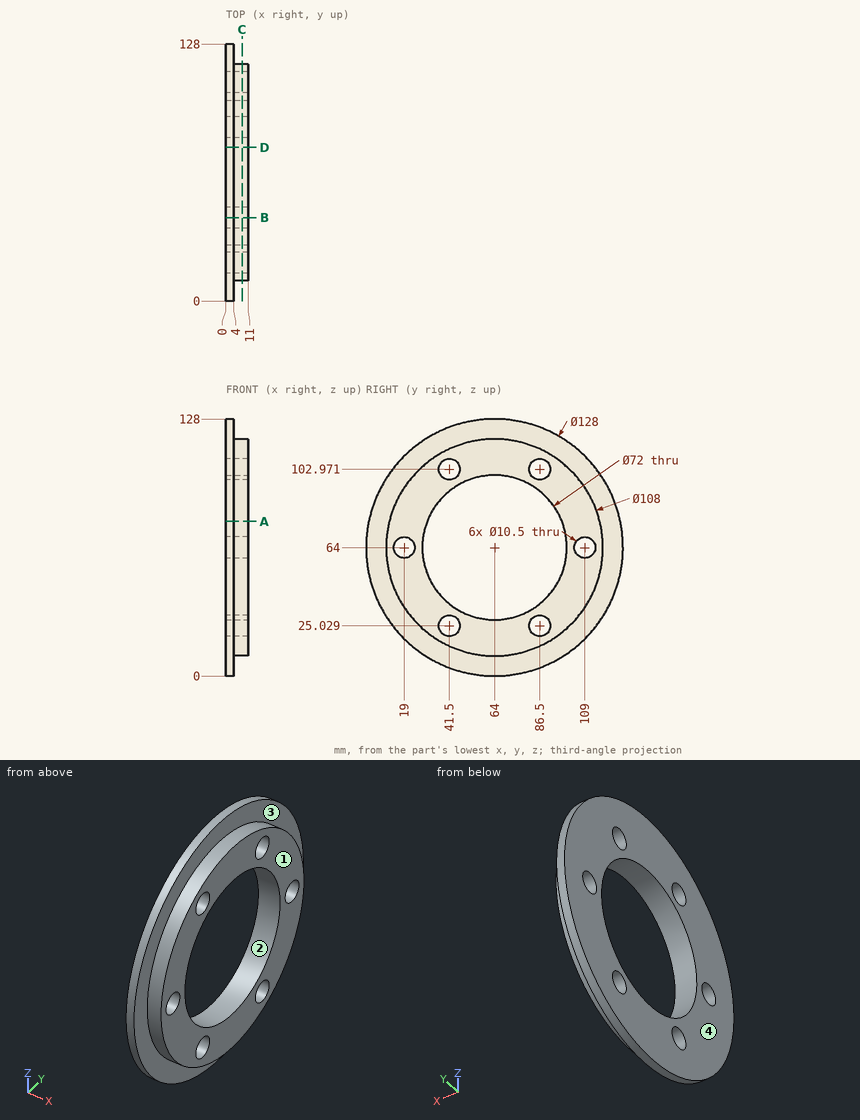
Job drawing, mm, ordinate dimensions from the low corner. One solid piece. A direction names the side the tool comes from. Give positions to 0.01 mm unless a question says otherwise; leave off trailing zeros. Loops run counter-clockwise (first coordinate to the right, second up) from the corner with the lowest first, then second, coordinate; pieces in that order, holes last.
Item 1: Slice it at C-C, the plane x = 8. List the corners of the cut face in (y, z).
Answers follow:
outline: circle Ø108 at (64, 64); hole circle Ø10.5 at (19, 64); hole circle Ø72 at (64, 64); hole circle Ø10.5 at (41.5, 25.03); hole circle Ø10.5 at (41.5, 102.97); hole circle Ø10.5 at (86.5, 25.03); hole circle Ø10.5 at (86.5, 102.97); hole circle Ø10.5 at (109, 64)
Item 2: Slice it at B-B, the plane y = 41.5. List the corners of the cut face in (x, z).
Answers follow:
outline: (0, 4.09) - (4, 4.09) - (4, 14.91) - (11, 14.91) - (11, 19.78) - (0, 19.78) - close; (0, 30.28) - (11, 30.28) - (11, 35.9) - (0, 35.9) - close; (0, 92.1) - (11, 92.1) - (11, 97.72) - (0, 97.72) - close; (0, 108.22) - (11, 108.22) - (11, 113.09) - (4, 113.09) - (4, 123.91) - (0, 123.91) - close
Item 3: Flat gauge pins, fed straight in: pin 1 (2 mm diameter, centred on x = 3.5, y = 80, fed in from -Z); pin 2 (1.5 mm diameter, centred on x = 9, z = 65, fed in from -Y); pin 3 (2 mm diameter, centred on x = 2.5, z = 21.5, fed in from +Y); pin 4 (6.5 mm diameter, centred on y = 109, z = 64, fed in from -X). Where does each tip first touch, or does it go through?
Answers follow:
pin 1: stops at z = 1.78
pin 2: stops at y = 10
pin 3: stops at y = 112.72
pin 4: passes through
Item 4: Drill centre lines: line 1 (Y direction, x = 3.75, z = 64); line 2 (Y direction, x = 6, z = 64); line 3 (Z direction, x = 3.75, y = 45) (1 decimal). Where is each one in solid material? Low to high.
Answers follow:
line 1: y = 0 to 13.75, 24.25 to 28, 100 to 103.75, 114.25 to 128
line 2: y = 10 to 13.75, 24.25 to 28, 100 to 103.75, 114.25 to 118
line 3: z = 2.9 to 21.1, 28.9 to 33.4, 94.6 to 99.1, 106.9 to 125.1
Item 5: Slice it at D-D, the plane y = 76.5. List the corners of the cut face in (x, z), and give its area (3 significant figures).
Answers follow:
outline: (0, 1.23) - (4, 1.23) - (4, 11.47) - (11, 11.47) - (11, 30.24) - (0, 30.24) - close; (0, 97.76) - (11, 97.76) - (11, 116.53) - (4, 116.53) - (4, 126.77) - (0, 126.77) - close
area: 495 mm2
Item 6: Slice it at A-A, the plane z = 77. List the corners of the cut face in (x, y).
Answers follow:
outline: (0, 1.33) - (4, 1.33) - (4, 11.59) - (11, 11.59) - (11, 30.43) - (0, 30.43) - close; (0, 97.57) - (11, 97.57) - (11, 116.41) - (4, 116.41) - (4, 126.67) - (0, 126.67) - close
Item 7: Pull direction Y, two halves, no side cores. Call the marked faces 1 and 2: released by +Y, released by -Y, zero draft, split by the parting line, or undercut.
Answers follow:
face 1: zero draft
face 2: undercut
Item 8: Which spindle directions (+Z, -Z, +X, -X, +Y, -Y) get a long thin tool onto all of the face, cutting with end or side? Do the marked faces 3 and 4. Say none if no direction does.
Answers follow:
face 3: +X
face 4: +Z, -Z, -X, +Y, -Y
